Autodesk Inventor part; units mm, degrees
ref_plane "YZ Plane" through (0, 0, 0) normal (1, 0, 0) x (0, 1, 0)
ref_plane "XZ Plane" through (0, 0, 0) normal (0, 1, 0) x (-1, 0, 0)
ref_plane "XY Plane" through (0, 0, 0) normal (0, 0, 1) x (1, 0, 0)
sketch "Sketch1" plane through (0, 0, 0) normal (0, 0, 1) x (1, 0, 0)
  line L0 (22.225, 0) -> (22.225, 3.175)
  line L1 (22.225, -47.625) -> (22.225, -44.45)
  line L2 (22.225, -44.45) -> (34.925, -44.45)
  line L3 (34.925, -44.45) -> (34.925, -47.625)
  line L4 (34.925, -47.625) -> (79.375, -47.625)
  line L5 (79.375, -47.625) -> (79.375, -44.45)
  line L6 (79.375, -44.45) -> (92.075, -44.45)
  line L7 (92.075, -44.45) -> (92.075, -47.625)
  line L8 (117.475, 3.175) -> (92.075, 3.175)
  line L9 (92.075, 3.175) -> (92.075, 0)
  line L10 (92.075, 0) -> (79.375, 0)
  line L11 (79.375, 0) -> (79.375, 3.175)
  line L12 (79.375, 3.175) -> (34.925, 3.175)
  line L13 (34.925, 3.175) -> (34.925, 0)
  line L14 (34.925, 0) -> (22.225, 0)
  line L15 (85.6063, -21.2725) -> (72.708, -21.2725)
  line L16 (72.708, -21.2725) -> (71.1205, -19.685)
  line L17 (71.1205, -19.685) -> (71.1205, -10.4775)
  line L18 (71.1205, -10.4775) -> (72.708, -8.89)
  line L19 (72.708, -8.89) -> (85.6063, -8.89)
  line L20 (85.6063, -8.89) -> (87.1938, -10.4775)
  line L21 (87.1938, -10.4775) -> (87.1938, -19.685)
  line L22 (87.1938, -19.685) -> (85.6063, -21.2725)
  line L23 (0, 0) -> (0, 3.175)
  line L24 (0, 3.175) -> (22.225, 3.175)
  line L25 (0, -27.6225) -> (-3.175, -27.6225)
  line L26 (-3.175, -27.6225) -> (-3.175, -14.9225)
  line L27 (-3.175, -14.9225) -> (0, -14.9225)
  line L28 (3.175, -14.9225) -> (3.175, -27.6225)
  line L29 (3.175, -27.6225) -> (-3.175, -14.9225) construction
  line L30 (-3.175, -27.6225) -> (3.175, -14.9225) construction
  line L31 (0, -47.625) -> (0, -27.6225)
  line L32 (0, -14.9225) -> (0, 3.175)
  line L33 (114.3, 0) -> (114.3, 3.175)
  line L34 (92.075, -47.625) -> (114.3, -47.625)
  line L35 (114.3, -28.575) -> (117.475, -28.575)
  line L36 (117.475, -28.575) -> (117.475, -15.875)
  line L37 (117.475, -15.875) -> (114.3, -15.875)
  line L38 (111.125, -15.875) -> (111.125, -28.575)
  line L39 (111.125, -28.575) -> (117.475, -15.875) construction
  line L40 (117.475, -28.575) -> (111.125, -15.875) construction
  line L41 (114.3, -47.625) -> (114.3, -28.575)
  line L42 (114.3, -15.875) -> (114.3, 3.175)
  line L43 (22.225, -47.625) -> (0, -47.625)
  point P0 (0, -21.2725)
  point P1 (114.3, -22.225)
  dimension "d2" = 6.35
  dimension "d3" = 12.7
  dimension "d4" = 6.35
  dimension "d5" = 12.7
extrude "Extrusion1" add sketch "Sketch1" along normal blind 3.175
properties part number "Side 2" material "ABS Plastic"
Could you check a few things on this model? Use its own coordinates, in mm. A direction names the side the tool comes from. Round coordinates to 2 decimals unless told otherwise and drop trailing zeros. Write each loop counter-clockwise with the first axis right and the second up, starting at its lowest first coordinate (ties: lowest second). Pieces come first, ordered by that corner, then holes. Notation, with made-up numbers: M -4,25.25 L 48,25.25 A21 ccw 48,35.25 Z; hole C 28.25,89 d10. An arc over 180 degrees is marked long. Answer in a Markdown table with one row per item. Add a question column.
Q1. Will these pins go through, and if not, where does the flat tip stop? pin 1 Ø1.5 at (y, z) = (-39.5, 1) entering from -X; pin 2 Ø1.6 at (y, z) = (-40.5, 2) entering from +X; pin 3 Ø1 at (x, z) = (85, 1) entering from +Y.
Q2. If we mould it in two halves opening along X, with no side actions, what happens to faces 1 (the flat face through (-3.175, -21, 2)), 2 (the flat face through (92.075, 2, 2)), 3 (the flat face through (114.3, -38, 2)), 4 (the flat face through (79.375, 2, 2))? For each: +X half, -X half, draft (parallel to the pull), parting line (faces both ways), or undercut.
Q3. If I drill on line 1 (Y direction, x = 83, z = 2.4); line 2 (X direction, y = -11.5, z = 2.75); line 3 (Y direction, x = 78.5, z = 1.65) (1 decimal), over which ranges is the centre line in solid material (lowest first)? Write a range as from..to.
Q4. Imagine slicing it at C-C (x = 24). Please give me the cut outline in (y, z) (3 decimals), then the cut area to 3 significant figures.
Q5. On a 3-axis mill with a long thin cutter (end or side, diameter ignored), from which of +Z, -Z, +X, -X, +Y, -Y can I reach the whole of each face in a straight line? I mean faces 5 (the flat face through (116, -28.575, 2)), 6 (the flat face through (28, -44.45, 2)), 7 (the flat face through (86, 0, 2)), 8 (the flat face through (71.12, -15, 2)), 9 (the flat face through (116, -15.875, 2)). Say none if no direction works.
Q6. Imagine slicing it at B-B (y = -39). Please give me the cut outline in (x, z) (3 decimals), then the cut area to 3 significant figures.
Q7. Imagine slicing it at A-A (x = 76.5). Please give me the cut outline in (y, z) (1 decimal).
Values:
| question | item | result |
|---|---|---|
| 1 | pin 1 | x = 0 |
| 1 | pin 2 | x = 114.3 |
| 1 | pin 3 | y = 0 |
| 2 | face 1 | -X half |
| 2 | face 2 | undercut |
| 2 | face 3 | +X half |
| 2 | face 4 | undercut |
| 3 | line 1 | -44.45..-21.27, -8.89..0 |
| 3 | line 2 | 0..71.12, 87.19..114.3 |
| 3 | line 3 | -47.6..-21.3, -8.9..3.2 |
| 4 | outline | M -44.45,0 L 0,0 L 0,3.175 L -44.45,3.175 Z |
| 4 | area | 141 mm^2 |
| 5 | face 5 | +Z, -Z, +X, -Y |
| 5 | face 6 | +Z, -Z, -Y |
| 5 | face 7 | +Z, -Z, +Y |
| 5 | face 8 | +Z, -Z |
| 5 | face 9 | +Z, -Z, +X, +Y |
| 6 | outline | M 0,0 L 114.3,0 L 114.3,3.175 L 0,3.175 Z |
| 6 | area | 363 mm^2 |
| 7 | outline | M -47.6,0 L -21.3,0 L -21.3,3.2 L -47.6,3.2 Z; M -8.9,0 L 3.2,0 L 3.2,3.2 L -8.9,3.2 Z |
